from build123d import *

# Parameters (mm, degrees)
SKETCH_W  = 5
SKETCH_H  = 20
PAD_DEPTH = 5


with BuildPart() as part:
    # Sketch → Pad (new body)
    with BuildSketch(Plane.XY):
        Polygon((74.918265, 123.488459), (74.918265, -126.511541), (-75.081735, -126.511541), (-75.081735, 123.488459), (-60.081735, 123.488459), (-60.081735, 93.488459), (-55.081735, 93.488459), (-55.081735, 123.488459), (-2.581735, 123.488459), (-2.581735, 93.488459), (2.418265, 93.488459), (2.418265, 123.488459), (54.918265, 123.488459), (54.918265, 93.488459), (59.918265, 93.488459), (59.918265, 123.488459), align=None)
        with Locations((-37.581735, -16.511541)):
            Rectangle(SKETCH_W, SKETCH_H, mode=Mode.SUBTRACT)
        with Locations((-37.581735, 18.488459)):
            Rectangle(SKETCH_W, SKETCH_H, mode=Mode.SUBTRACT)
        with Locations((-37.581735, 53.488459)):
            Rectangle(SKETCH_W, SKETCH_H, mode=Mode.SUBTRACT)
        with Locations((-37.581735, -51.511541)):
            Rectangle(SKETCH_W, SKETCH_H, mode=Mode.SUBTRACT)
        with Locations((-37.581735, -86.511541)):
            Rectangle(SKETCH_W, SKETCH_H, mode=Mode.SUBTRACT)
        with Locations((57.418265, -16.511541)):
            Rectangle(SKETCH_W, SKETCH_H, mode=Mode.SUBTRACT)
        with Locations((57.418265, -51.511541)):
            Rectangle(SKETCH_W, SKETCH_H, mode=Mode.SUBTRACT)
        with Locations((57.418265, -86.511541)):
            Rectangle(SKETCH_W, SKETCH_H, mode=Mode.SUBTRACT)
        with Locations((57.418265, 18.488459)):
            Rectangle(SKETCH_W, SKETCH_H, mode=Mode.SUBTRACT)
        with Locations((57.418265, 53.488459)):
            Rectangle(SKETCH_W, SKETCH_H, mode=Mode.SUBTRACT)
    extrude(amount=PAD_DEPTH)


solid = part.part
CAD build for the part. Positions are in the model's coordinates, mm. A direction names the side the tool comes from. Coordinates: 2 decimals unless noted, no trailing zeros. Loops run counter-clockwise (first coordinate to the right, second up) from the corner with the lowest first, then second, coordinate; pieces in that order, holes last. Notation, with made-up numbers: (88.5, -31.5) - (105.5, -31.5) arc R16 cw to (105.5, -15.5) - close; hole circle Ø8 at (-20.75, 9.25). An arc over 180 degrees is marked (long way). Write item = value, one per line. Start each with the question number.
Q1. Cut at B-B, the plane z = 1.55. Give the number of separate pieces and of enclosed holes in the cut face, then the cut area to 4 significant figures.
Q2. Which spindle directions (+Z, -Z, +X, -X, +Y, -Y) get a long thin tool onto all of the face, cutting with end or side? Do faces 1 (the flat face through (57, 93.488, 2)), 2 (the flat face through (74.918, 0, 2)), 3 (the flat face through (-38, 8.488, 2)). Say none if no direction does.
Q3. Pull direction Y, two halves, no side cores. Call faces 4 (the flat face through (-35.082, -52, 2)), 5 (the flat face through (1, -126.512, 2)), 6 (the flat face through (-2.582, 109, 2)), 7 (the flat face through (0, 93.488, 2)): pulls with the +Y half, pulls with the -Y half, needs draft (parallel to the pull), parting line crosses it, or undercut.
Q4. Flat gauge pin, fed straight in: pin 1 Ø1.5 at (x, z) = (58, 1.5) entering from +Y. Where does the tip first touch, or does it go through?
Q5. Cut at A-A, the plane y = 46.5. List the corners of the cut face in (x, z).
Q6. Drill centre lines: L1, parallel to X at y = 46, z = 0.8; L2, parallel to Y at x = 57.5, z = 0.6; L3, parallel to X at y = 110, z = 3.9. Where is each one in solid material? Low to high.
Computed:
q1.separate_pieces = 1
q1.enclosed_holes = 10
q1.area = 36,050 mm²
q2.face_1 = +Z, -Z, +Y
q2.face_2 = +Z, -Z, +X, +Y, -Y
q2.face_3 = +Z, -Z
q3.face_4 = undercut
q3.face_5 = pulls with the -Y half
q3.face_6 = needs draft
q3.face_7 = pulls with the +Y half
q4.pin_1 = 93.49
q5.outline = (-75.08, 0) - (-40.08, 0) - (-40.08, 5) - (-75.08, 5) - close; (-35.08, 0) - (54.92, 0) - (54.92, 5) - (-35.08, 5) - close; (59.92, 0) - (74.92, 0) - (74.92, 5) - (59.92, 5) - close
q6.L1 = -75.08 to -40.08, -35.08 to 54.92, 59.92 to 74.92
q6.L2 = -126.51 to -96.51, -76.51 to -61.51, -41.51 to -26.51, -6.51 to 8.49, 28.49 to 43.49, 63.49 to 93.49
q6.L3 = -75.08 to -60.08, -55.08 to -2.58, 2.42 to 54.92, 59.92 to 74.92
